Here's how the part is built. I have some questions about the finished solid (model axes, mm). A direction names the side the tool comes from. Coordinates: 2 decimals unless noted, no trailing zeros. Loops run counter-clockwise (first coordinate to the right, second up) from the corner with the lowest first, then second, coordinate; pieces in that order, holes last. Notation, with made-up numbers: M -3,-1.75 L 56,-1.75 A28 cw 56,24.25 Z; hole C 31.5,50 d5. An arc over 180 degrees is marked long. Use CSV: the item, a comma, the result in double quotes. Start each with the question number.
Q1. If we section it at A-A (y = 12.25): Please give me the cut outline in (x, z).
Q2. Please list where these lines run through material, in increasing order: probe 1 along Z at (x, y) = (-20, 20.6); probe 2 along Y at (x, z) = (38, 17); probe 3 along X at (y, z) = (13.5, 11). Write a range as [from, to].
Q3. If we mould it in two halves opening along Y, with no side actions, what happens to faces 1 (the flat face through (-1, 21.5, -1)), 2 (the cylindrical face through (-30.843, 20.74, 29.411)), 3 (the flat face through (-5, 15, 0))? For each: +Y half, -Y half, draft (parallel to the pull), parting line (faces both ways), or undercut.
Q4. If we section it at D-D (x = -20): Please give me the cut outline in (y, z), and give its area (3 significant figures).
Q5. For pin 1 Ø4 at (x, z) = (36, -20.5) entering from -Y; pin 2 Ø1.5 at (x, y) = (20.5, 18) entering from +Z; pin 3 Ø12 at (x, z) = (13, -7) entering from -Y, each with a flat end and sliding along its axis, tell me the tip position at first contact or that it passes through.
Q6. Which directions (+Z, -Z, +X, -X, +Y, -Y) give clear straight access to the entire face, cutting with the end or side of a thin tool? Please do faces 4 (the flat face through (0, 9, 20)), 5 (the cylindrical face through (-21.39, 20.76, 40.06)), 6 (the flat face through (0, 9, -20)), 7 (the flat face through (5, 15, 0)).
Q7. If we section it at C-C (x = 4.5): Please give me the cut outline in (y, z), and give its area (3 significant figures).
Q8. If we section it at B-B (z = 0): Please give me the cut outline in (x, y), and give its area (3 significant figures).
Autodesk Inventor part; units mm, degrees
ref_plane "Work Plane3" through (-4.3301, 20, -20) normal (0, 1, 0) x (1, 0, 0)
ref_plane "Work Plane2" through (0, 21.5, 0) normal (0, 1, 0) x (1, 0, 0)
ref_plane "YZ Plane" through (0, 0, 0) normal (1, 0, 0) x (0, 1, 0)
ref_plane "Work Plane3" through (-4.3301, 20, -20) normal (0, 1, 0) x (1, 0, 0)
sketch "Sketch4" plane through (-4.3301, 20, -20) normal (0, 1, 0) x (1, 0, 0)
  circle A0 centre (4.3301, -20) radius 50
  dimension "d16" = 100
extrude "Extrusion4" add sketch "Sketch4" along normal blind 1.5
sketch "Sketch9" plane through (0, 0, 0) normal (0, 0, 1) x (1, 0, 0)
  line L0 (50, 21.5) -> (-50, 21.5)
  line L1 (50, 21.5) -> (43, 21.5)
  line L2 (50, 21.5) -> (50, 26.5)
  line L3 (50, 26.5) -> (48, 26.5)
  line L4 (48, 26.5) -> (43, 21.5)
  line L5 (0, 21.5) -> (0, 37.2)
  point P0 (0, 0)
  dimension "d27" = 7
  dimension "d28" = 5
  dimension "d29" = 2
revolve "Revolution1" add sketch "Sketch9" angle 360 about axis through (0, 21.5, 0) along (0, 1, 0)
ref_plane "Work Plane2" through (0, 21.5, 0) normal (0, 1, 0) x (1, 0, 0)
sketch "Sketch12" plane through (0, 21.5, 0) normal (0, 1, 0) x (1, 0, 0)
  line L0 (0, 0) -> (20, 0)
  line L1 (20, 0) -> (20, -35)
  line L2 (20, -35) -> (-20, -35)
  line L3 (-20, -35) -> (-20, 35)
  line L4 (-20, 35) -> (20, 35)
  line L5 (20, 35) -> (20, -35)
  circle A0 centre (20, 35) radius 1.75
  circle A1 centre (-20, 35) radius 1.75
  circle A2 centre (-20, -35) radius 1.75
  circle A3 centre (20, -35) radius 1.75
  dimension "d47" = 20
  dimension "d48" = 35
  dimension "d49" = 40
  dimension "d50" = 70
  dimension "d51" = 3.5
  dimension "d52" = 3.5
  dimension "d53" = 3.5
  dimension "d54" = 3.5
extrude "Extrusion6" cut sketch "Sketch12" against normal blind 1.5 contours A3 L2 L1 | L1 L2 A3 | A0 L4 L5 | L5 L4 A0 | A2 L3 L2 | L2 L3 A2 | A1 L3 L4 | L4 L3 A1
sketch "Sketch13" plane through (0, 0, 0) normal (0, 0, 1) x (1, 0, 0)
  line L0 (0, 0) -> (25, 0) construction
  line L1 (-50, 20) -> (50, 20)
  line L2 (0, 7.5) -> (-21.6506, 20)
  line L3 (0, 7.5) -> (21.6506, 20)
  line L4 (0, 7.5) -> (25, 7.5) construction
  line L5 (21.6506, 20) -> (-21.6506, 20)
  line L6 (0, 7.5) -> (0, 12.5)
  line L7 (0, 20) -> (-5, 20)
  line L8 (-5, 20) -> (0, 12.5)
  line L9 (0, 20) -> (5, 20)
  line L10 (5, 20) -> (0, 12.5)
  dimension "d60" = 25
  dimension "d61" = 30
  dimension "d62" = 5
  dimension "d63" = 5
  dimension "d64" = 5
extrude "Extrusion7" add sketch "Sketch13" along normal mid plane 40 contours L1 L8 L6 L2 | L6 L10 L1 L3
sketch "Sketch16" plane through (0, 0, 20) normal (0, 0, 1) x (1, 0, 0)
  line L0 (-50, 20) -> (50, 20)
  line L1 (0, 20) -> (0, 5)
  line L2 (0, 5) -> (23.8952, 18.7959)
  line L3 (23.8952, 18.7959) -> (25.9808, 20)
  line L4 (25.9808, 20) -> (-25.9812, 20)
  line L5 (-25.9812, 20) -> (0, 5)
  point P0 (0, 0)
  dimension "d67" = 15
  dimension "d68" = 60
  dimension "d69" = 51.962
extrude "Extrusion8" add sketch "Sketch16" against normal blind 40
sketch "Sketch17" plane through (0, 0, 20) normal (0, 0, 1) x (1, 0, 0)
  line L0 (0, 5) -> (-25.9812, 20)
  line L1 (0, 5) -> (0, 10)
  line L2 (0, 10) -> (6.8298, 16.8298)
  line L3 (6.8298, 16.8298) -> (10, 20)
  line L4 (-50, 20) -> (50, 20)
  line L5 (10, 20) -> (-10, 20)
  line L6 (-10, 20) -> (0, 10)
  point P0 (0, 0)
  dimension "d72" = 5
  dimension "d73" = 135
  dimension "d74" = 20
extrude "Extrusion9" cut sketch "Sketch17" against normal blind 40 contours L6 L4 L3 L2
sketch "Sketch18" plane through (0, 20, 0) normal (0, -1, 0) x (1, 0, 0)
  line L0 (0, 0) -> (-35.3553, 35.3553)
  circle A0 centre (0, 0) radius 50
  line L1 (0, 0) -> (50, 0) construction
  line L2 (0, 0) -> (35.3553, 35.3553)
  line L3 (0, 0) -> (50, 0) construction
  line L4 (0, 0) -> (-35.3553, -35.3553)
  line L5 (0, 0) -> (50, 0) construction
  line L6 (0, 0) -> (35.3553, -35.3553)
  line L7 (0, 0) -> (50, 0) construction
  circle A1 centre (0, 0) radius 43
  line L8 (-30.4056, 30.4056) -> (-29.3449, 29.3449)
  line L9 (30.4056, 30.4056) -> (29.3449, 29.3449)
  line L10 (30.4056, -30.4056) -> (29.3449, -29.3449)
  line L11 (-30.4056, -30.4056) -> (-29.3449, -29.3449)
  circle A2 centre (-29.3449, -29.3449) radius 1.5
  circle A3 centre (29.3449, -29.3449) radius 1.5
  circle A4 centre (-29.3449, 29.3449) radius 1.5
  circle A5 centre (29.3449, 29.3449) radius 1.5
  dimension "d77" = 135
  dimension "d78" = 45
  dimension "d79" = 135
  dimension "d80" = 45
  dimension "d81" = 1.5
  dimension "d82" = 1.5
  dimension "d83" = 1.5
  dimension "d84" = 1.5
extrude "Extrusion10" cut sketch "Sketch18" against normal blind 40 contours A4 L0 | L0 A4 | A5 L2 | L2 A5 | A2 L4 | L4 A2 | A3 L6 | L6 A3
sketch "Sketch20" plane through (-4.3301, 21.5, -20) normal (0, 1, 0) x (1, 0, 0)
  circle A0 centre (-15.6699, 15) radius 1.75
  circle A1 centre (-15.6699, 15) radius 3.5
  circle A2 centre (24.3301, 15) radius 1.75
  circle A3 centre (24.3301, 15) radius 3.5
  circle A4 centre (24.3301, -55) radius 1.75
  circle A5 centre (24.3301, -55) radius 3.5
  circle A6 centre (-15.6699, -55) radius 1.75
  circle A7 centre (-15.6699, -55) radius 3.5
  point P0 (4.3301, -20)
  dimension "d87" = 7
  dimension "d88" = 7
  dimension "d89" = 7
  dimension "d90" = 7
extrude "Extrusion11" cut sketch "Sketch20" along normal blind 10
sketch "Sketch21" plane through (-4.3301, 21.5, -20) normal (0, 1, 0) x (1, 0, 0)
  circle A0 centre (4.3301, -20) radius 67.7461
extrude "Extrusion12" cut sketch "Sketch21" along normal blind 10
sketch "Sketch22" plane through (0, 5, -20) normal (0.5, -0.866, 0) x (0.866, 0.5, 0)
  point P0 (-2.5, 20)
sketch "Sketch23" plane through (0, 21.5, 0) normal (0, 1, 0) x (1, 0, 0)
  circle A0 centre (20, -35) radius 1.75
  line L0 (20, -35) -> (20, -39)
  circle A1 centre (-20, -35) radius 1.75
  line L1 (-20, -35) -> (-20, -39)
  circle A2 centre (20, -39) radius 1.75
  circle A3 centre (-20, -39) radius 1.75
  point P0 (0, 0)
  dimension "d95" = 4
  dimension "d96" = 4
  dimension "d97" = 3.5
  dimension "d98" = 3.5
extrude "Extrusion13" cut sketch "Sketch23" against normal blind 10 contours A2 | A3
sketch "Sketch24" plane through (0, 21.5, 0) normal (0, 1, 0) x (1, 0, 0)
  circle A0 centre (20, -35) radius 1.75
  circle A1 centre (20, -35) radius 1.75
  circle A2 centre (-20, -35) radius 1.75
  circle A3 centre (-20, -35) radius 1.75
  point P0 (0, 0)
extrude "Extrusion14" add sketch "Sketch24" against normal blind 1.5
properties part number "Mirror Mount" material "Acetal Resin, Black"
Results below:
1,outline,"M -12.56,-20 L -2.25,-20 L -2.25,20 L -12.56,20 Z; M 2.25,-20 L 12.56,-20 L 12.56,20 L 2.25,20 Z"
2,probe 1,"[-45.83, -36.75], [-33.25, 37.25], [40.75, 45.83]"
2,probe 2,"[20, 21.5]"
2,probe 3,"[-14.72, -3.5], [3.5, 14.72]"
3,face 1,"+Y half"
3,face 2,"draft"
3,face 3,"undercut"
4,outline,"M 16.55,-20 L 20,-20 L 20,-33.25 L 21.5,-33.25 L 21.5,37.25 L 20,37.25 L 20,20 L 16.55,20 Z; M 20,-45.83 L 21.5,-45.83 L 21.5,-36.75 L 20,-36.75 Z; M 20,40.75 L 21.5,40.75 L 21.5,45.83 L 20,45.83 Z"
4,area,"265 mm^2"
5,pin 1,"y = 20"
5,pin 2,"z = 20"
5,pin 3,"y = 9.04"
6,face 4,"+Z, +X, -X, -Y"
6,face 5,"+Y, -Y"
6,face 6,"-Z, +X, -X, -Y"
6,face 7,"+Z, -Z"
7,outline,"M 7.6,-20 L 14.5,-20 L 14.5,20 L 7.6,20 Z; M 20,-49.8 L 21.5,-49.8 L 21.5,49.8 L 20,49.8 Z"
7,area,"425 mm^2"
8,outline,"M -50,20 L -25.98,20 L 0,5 L 23.9,18.8 L 25.98,20 L 50,20 L 50,21.5 L -50,21.5 Z; hole M -10,20 L 0,10 L 10,20 Z"
8,area,"440 mm^2"
